Read the model definition and answer for the solid it produces. Units are mm, in the model's axes. Face numbers are marked on the shaded views. A direction names the side the tool comes from. Give positions to 0.01 mm unless a question says otherwise; leave off trailing zeros. Write each loop counter-clockwise with the first axis right and the second up, starting at its lowest first coordinate (ties: lowest second). Pieces come first, ordered by that corner, then holes.
Autodesk Inventor part; units mm, degrees
ref_plane "YZ Plane" through (0, 0, 0) normal (1, 0, 0) x (0, 1, 0)
ref_plane "XZ Plane" through (0, 0, 0) normal (0, 1, 0) x (-1, 0, 0)
ref_plane "XY Plane" through (0, 0, 0) normal (0, 0, 1) x (1, 0, 0)
sketch "スケッチ1" plane through (0, 0, 0) normal (0, 0, 1) x (1, 0, 0)
  line L0 (0, 0) -> (9, 0)
  line L1 (9, 0) -> (9, -9)
  line L2 (9, -9) -> (0, -9)
  line L3 (0, -9) -> (0, 0)
  line L4 (1.2, -1.2) -> (7.8, -1.2)
  line L5 (7.8, -1.2) -> (7.8, -7.8)
  line L6 (7.8, -7.8) -> (1.2, -7.8)
  line L7 (1.2, -7.8) -> (1.2, -1.2)
  dimension "d0" = 9
  dimension "d1" = 9
  dimension "d2" = 1.2
  dimension "d3" = 1.2
  dimension "d4" = 1.2
  dimension "d5" = 1.2
extrude "押し出し1" add sketch "スケッチ1" along normal blind 44
sketch "スケッチ2" plane through (0, 0, 0) normal (0, 1, 0) x (1, 0, 0)
  line L0 (0, 0) -> (0, -44)
  line L1 (9, 0) -> (0, 0)
  line L2 (0, -44) -> (9, -44)
  point P0 (4.5, -39.5)
  point P1 (4.5, -4.5)
  dimension "d8" = 4.5
  dimension "d26" = 4.5
  dimension "d27" = 4.5
  dimension "d28" = 4.5
hole "穴1" at (4.5, 0, 39.5) at (4.5, 0, 4.5) direction (0, -1, 0) diameter 3.3 end through all
sketch "スケッチ3" plane through (9, -9, 0) normal (1, 0, 0) x (0, 0, -1)
  line L0 (-44, 0) -> (-44, 9)
  line L1 (0, 9) -> (-44, 9)
  line L2 (0, 0) -> (0, 9)
  point P0 (-30.5, 4.5)
  point P1 (-13.5, 4.5)
  dimension "d17" = 13.5
  dimension "d18" = 4.5
  dimension "d29" = 13.5
  dimension "d30" = 4.5
hole "穴2" at (9, -4.5, 30.5) at (9, -4.5, 13.5) direction (-1, 0, 0) diameter 3.3 end through all
sketch "スケッチ4" plane through (0, -9, 0) normal (0, -1, 0) x (1, 0, 0)
  line L0 (9, 0) -> (9, 44)
  circle A0 centre (4.5, 39.5) radius 1.65
  point P0 (0, 0)
  point P1 (4.5, 34.5)
  point P2 (4.5, 29.5)
  point P3 (4.5, 24.5)
  point P4 (4.5, 19.5)
  point P5 (4.5, 14.5)
  point P6 (4.5, 9.5)
  dimension "d31" = 4.5
  dimension "d32" = 5
  dimension "d35" = 5
hole "穴3" at (4.5, -9, 34.5) at (4.5, -9, 29.5) at (4.5, -9, 24.5) at (4.5, -9, 19.5) at (4.5, -9, 14.5) at (4.5, -9, 9.5) direction (0, 1, 0) diameter 4 end through all
sketch "スケッチ5" plane through (0, -9, 0) normal (-1, 0, 0) x (0, 0, 1)
  circle A0 centre (13.5, 4.5) radius 1.65
  line L0 (0, 9) -> (0, 0)
  line L1 (44, 9) -> (44, 0)
  line L2 (0, 9) -> (44, 9)
  circle A1 centre (30.5, 4.5) radius 1.65
  point P0 (6.75, 4.5)
  point P1 (37.25, 4.5)
  point P2 (22, 4.5)
  dimension "d47" = 13.5
  dimension "d48" = 6.75
  dimension "d49" = 6.75
  dimension "d50" = 4.5
  dimension "d51" = 4.5
  dimension "d52" = 4.5
  dimension "d53" = 17
  dimension "d54" = 8.5
hole "穴4" at (0, -4.5, 6.75) at (0, -4.5, 37.25) at (0, -4.5, 22) direction (1, 0, 0) diameter 5 end through all
equation "\"d3\" = d2"
equation "\"d4\" = d3"
equation "\"d5\" = d2"
properties part number "ハンド9x9_2" material "アルミニウム 6061"
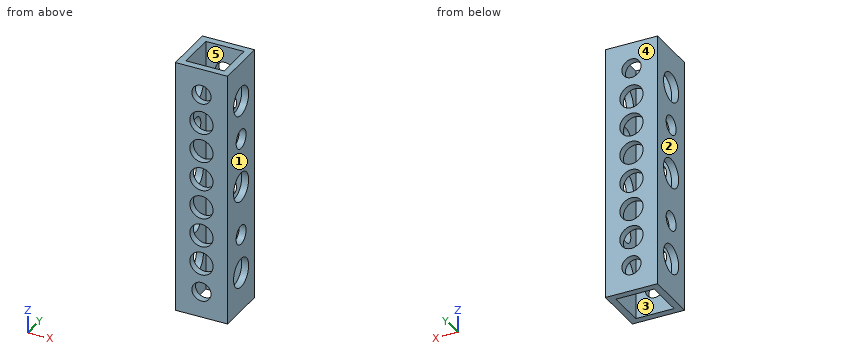
Item 1: Find the intervals of material crossed by line 1 along Z through (x, y) = (0.9, -4.5); line 2 along Y through (x, z) = (2.25, 26); line 3 along Y through (x, z) = (0.75, 13.5), in increasing order.
Result set:
line 1: z = 0 to 4.25, 9.25 to 11.85, 15.15 to 19.5, 24.5 to 28.85, 32.15 to 34.75, 39.75 to 44
line 2: y = -9 to -7.8, -1.2 to 0
line 3: y = -9 to -6.15, -2.85 to 0
Item 2: Which of the six approach directions +Z, -Z, +X, -X, +Y, -Y give full straight-line access (tool end or side, diameter ignored) to the marked faces 4 and 5?
Result set:
face 4: +Z, -Z, +X, -X, +Y
face 5: +Z, -Z
Item 3: Section C-C (y = -4.5) is taken. Give the number of separate pieces and of enclosed holes in the cut face, and give its area (3 significant figures).
Result set:
separate pieces: 12
enclosed holes: 0
area: 53.8 mm2
Item 4: Determine the mould class of the marked faces 1, 2 and 3 for opening direction X: pulls with the +X half, pulls with the -X half, needs draft (parallel to the pull), parting line crosses it, or undercut.
Result set:
face 1: pulls with the +X half
face 2: pulls with the -X half
face 3: undercut
Item 5: Section A-A (z = 6.75) is taken. Write down the section's boundary in (x, y).
Result set:
outline: (0, -9) - (9, -9) - (9, -7) - (7.8, -7) - (7.8, -7.8) - (1.2, -7.8) - (1.2, -7) - (0, -7) - close; (0, -2) - (1.2, -2) - (1.2, -1.2) - (7.8, -1.2) - (7.8, -2) - (9, -2) - (9, 0) - (0, 0) - close
Item 6: Section B-B (z = 13.5) is taken. Write down the section's boundary in (x, y).
Result set:
outline: (0, -9) - (2.77, -9) - (2.77, -7.8) - (1.2, -7.8) - (1.2, -6.15) - (0, -6.15) - close; (0, -2.85) - (1.2, -2.85) - (1.2, -1.2) - (2.77, -1.2) - (2.77, 0) - (0, 0) - close; (6.23, -9) - (9, -9) - (9, -6.15) - (7.8, -6.15) - (7.8, -7.8) - (6.23, -7.8) - close; (6.23, -1.2) - (7.8, -1.2) - (7.8, -2.85) - (9, -2.85) - (9, 0) - (6.23, 0) - close
